Build history of the part. All positions in model axes, mm. A direction names the side the tool comes from. Round coordinates to 2 decimals unless told otherwise and drop trailing zeros. Write each loop counter-clockwise with the first axis right and the second up, starting at its lowest first coordinate (ties: lowest second). Pieces come first, ordered by that corner, then holes. Notation, with made-up numbers: (36.5, 28.5) -> (89.5, 28.5) arc R18 cw to (89.5, 38.5) -> close; hole circle Ø7 at (6.5, 3). An arc over 180 degrees is marked (long way). Answer in a Markdown table with one row per item. Add a question column.
from build123d import *

# Parameters (mm, degrees)
SKETCH1_R                = 88
BOSS_EXTRUDE3_DEPTH      = 25
SKETCH4_W                = 10.4719
SKETCH4_H                = 13.351164338
BOSS_EXTRUDE4_DEPTH      = 25
FILLET2_R                = 4
CIRPATTERN1_COUNT        = 30
FILLET2_OF_CIRPATTERN1_R = 4
SKETCH6_R                = 10
BOSS_EXTRUDE5_DEPTH      = 60
BOSS_EXTRUDE6_START      = 10
SKETCH7_R                = 10
BOSS_EXTRUDE6_DEPTH      = 10
SKETCH8_R                = 10
BOSS_EXTRUDE7_DEPTH      = 10
SKETCH9_R                = 10
BOSS_EXTRUDE8_DEPTH      = 25
SKETCH10_R               = 10
BOSS_EXTRUDE9_DEPTH      = 42.5
SKETCH12_R               = 12.5
CUT_EXTRUDE1_DEPTH       = 12
CUT_EXTRUDE2_START       = -55.5
SKETCH13_R               = 10
CUT_EXTRUDE2_DEPTH       = 55.5
SKETCH14_R               = 10
BOSS_EXTRUDE10_DEPTH     = 440
SKETCH15_R               = 105
BOSS_EXTRUDE12_DEPTH     = 25
BOSS_EXTRUDE13_START     = 30
SKETCH16_R               = 105
BOSS_EXTRUDE13_DEPTH     = 30
SKETCH17_R               = 10
BOSS_EXTRUDE14_DEPTH     = 50
SKETCH18_R               = 10
BOSS_EXTRUDE15_DEPTH     = 30
SKETCH19_R               = 105
SKETCH19_R_2             = 90
CUT_EXTRUDE3_DEPTH       = 100
SHELL3_START             = -30
SHELL3_OUTLINE_R         = 80
SHELL3_DEPTH             = 45
SCALE2_SCALE             = 0.2


# Read off the part's stored shape, not the designer's step: Shell3
with BuildPart() as part:
    # Sketch1 → Boss-Extrude3 (new body)
    with BuildSketch(Plane.XY):
        Circle(SKETCH1_R)
    extrude(amount=BOSS_EXTRUDE3_DEPTH)

    # Sketch4 → Boss-Extrude4 (add)
    with BuildSketch(Plane.XY.offset(25)):
        with Locations((0, 93.324417831)):
            Rectangle(SKETCH4_W, SKETCH4_H)
    boss_extrude4 = extrude(amount=-BOSS_EXTRUDE4_DEPTH)

    # Fillet2
    fillet2_edges = [part.edges().sort_by_distance(p)[0] for p in [
        (5.23595, 100, 12.5),
        (0, 100, 0),
        (-5.23595, 100, 12.5),
        (0, 100, 25),
    ]]
    fillet(fillet2_edges, radius=FILLET2_R)

    # CirPattern1: Boss-Extrude4 ×30 about axis
    cirpattern1_axis = Axis((0, 0.317667884, 0), (0, 0, 1))
    for i in range(1, CIRPATTERN1_COUNT):
        add(boss_extrude4.rotate(cirpattern1_axis, i * 360 / CIRPATTERN1_COUNT))

    # Fillet2 of CirPattern1
    fillet2_of_cirpattern1_edges = [part.edges().sort_by_distance(p)[0] for p in [
        (-15.603590285, 98.910317096, 12.5),
        (-20.725122215, 97.821701879, 0),
        (-25.846654145, 96.733086661, 12.5),
        (-20.725122215, 97.821701879, 25),
        (-35.7611788, 93.511662322, 12.5),
        (-40.544457139, 91.382009596, 0),
        (-45.327735478, 89.252356869, 12.5),
        (-40.544457139, 91.382009596, 25),
        (-54.3558322, 84.039982796, 12.5),
        (-58.591804732, 80.962368605, 0),
        (-62.827777264, 77.884754413, 12.5),
        (-58.591804732, 80.962368605, 25),
        (-70.574874905, 70.909236365, 12.5),
        (-74.078409304, 67.018167216, 0),
        (-77.581943702, 63.127098067, 12.5),
        (-74.078409304, 67.018167216, 25),
        (-83.709456921, 54.693299655, 12.5),
        (-86.327431921, 50.158833942, 0),
        (-88.945406921, 45.624368229, 12.5),
        (-86.327431921, 50.158833942, 25),
        (-93.185533987, 36.100886913, 12.5),
        (-94.803531519, 31.121202547, 0),
        (-96.42152905, 26.14151818, 12.5),
        (-94.803531519, 31.121202547, 25),
        (-98.588956064, 15.944575793, 12.5),
        (-99.136261871, 10.737308875, 0),
        (-99.683567678, 5.530041957, 12.5),
        (-99.136261871, 10.737308875, 25),
        (-99.683567678, -4.894706189, 12.5),
        (-99.136261871, -10.101973107, 0),
        (-98.588956064, -15.309240025, 12.5),
        (-99.136261871, -10.101973107, 25),
        (-96.42152905, -25.506182413, 12.5),
        (-94.803531519, -30.485866779, 0),
        (-93.185533987, -35.465551145, 12.5),
        (-94.803531519, -30.485866779, 25),
        (-88.945406921, -44.989032461, 12.5),
        (-86.327431921, -49.523498174, 0),
        (-83.709456921, -54.057963887, 12.5),
        (-86.327431921, -49.523498174, 25),
        (-77.581943702, -62.491762299, 12.5),
        (-74.078409304, -66.382831448, 0),
        (-70.574874905, -70.273900597, 12.5),
        (-74.078409304, -66.382831448, 25),
        (-62.827777264, -77.249418645, 12.5),
        (-58.591804732, -80.327032837, 0),
        (-54.3558322, -83.404647029, 12.5),
        (-58.591804732, -80.327032837, 25),
        (-45.327735478, -88.617021102, 12.5),
        (-40.544457139, -90.746673828, 0),
        (-35.7611788, -92.876326554, 12.5),
        (-40.544457139, -90.746673828, 25),
        (-25.846654145, -96.097750894, 12.5),
        (-20.725122215, -97.186366111, 0),
        (-15.603590285, -98.274981329, 12.5),
        (-20.725122215, -97.186366111, 25),
        (-5.23595, -99.364664232, 12.5),
        (0, -99.364664232, 0),
        (5.23595, -99.364664232, 12.5),
        (0, -99.364664232, 25),
        (15.603590285, -98.274981329, 12.5),
        (20.725122215, -97.186366111, 0),
        (25.846654145, -96.097750894, 12.5),
        (20.725122215, -97.186366111, 25),
        (35.7611788, -92.876326554, 12.5),
        (40.544457139, -90.746673828, 0),
        (45.327735478, -88.617021102, 12.5),
        (40.544457139, -90.746673828, 25),
        (54.3558322, -83.404647029, 12.5),
        (58.591804732, -80.327032837, 0),
        (62.827777264, -77.249418645, 12.5),
        (58.591804732, -80.327032837, 25),
        (70.574874905, -70.273900597, 12.5),
        (74.078409304, -66.382831448, 0),
        (77.581943702, -62.491762299, 12.5),
        (74.078409304, -66.382831448, 25),
        (83.709456921, -54.057963887, 12.5),
        (86.327431921, -49.523498174, 0),
        (88.945406921, -44.989032461, 12.5),
        (86.327431921, -49.523498174, 25),
        (93.185533987, -35.465551145, 12.5),
        (94.803531519, -30.485866779, 0),
        (96.42152905, -25.506182413, 12.5),
        (94.803531519, -30.485866779, 25),
        (98.588956064, -15.309240025, 12.5),
        (99.136261871, -10.101973107, 0),
        (99.683567678, -4.894706189, 12.5),
        (99.136261871, -10.101973107, 25),
        (99.683567678, 5.530041957, 12.5),
        (99.136261871, 10.737308875, 0),
        (98.588956064, 15.944575793, 12.5),
        (99.136261871, 10.737308875, 25),
        (96.42152905, 26.14151818, 12.5),
        (94.803531519, 31.121202547, 0),
        (93.185533987, 36.100886913, 12.5),
        (94.803531519, 31.121202547, 25),
        (88.945406921, 45.624368229, 12.5),
        (86.327431921, 50.158833942, 0),
        (83.709456921, 54.693299655, 12.5),
        (86.327431921, 50.158833942, 25),
        (77.581943702, 63.127098067, 12.5),
        (74.078409304, 67.018167216, 0),
        (70.574874905, 70.909236365, 12.5),
        (74.078409304, 67.018167216, 25),
        (62.827777264, 77.884754413, 12.5),
        (58.591804732, 80.962368605, 0),
        (54.3558322, 84.039982796, 12.5),
        (58.591804732, 80.962368605, 25),
        (45.327735478, 89.252356869, 12.5),
        (40.544457139, 91.382009596, 0),
        (35.7611788, 93.511662322, 12.5),
        (40.544457139, 91.382009596, 25),
        (25.846654145, 96.733086661, 12.5),
        (20.725122215, 97.821701879, 0),
        (15.603590285, 98.910317096, 12.5),
        (20.725122215, 97.821701879, 25),
    ]]
    fillet(fillet2_of_cirpattern1_edges, radius=FILLET2_OF_CIRPATTERN1_R)

    # Sketch6 → Boss-Extrude5 (add)
    with BuildSketch(Plane.XY.offset(25)):
        Circle(SKETCH6_R)
    extrude(amount=BOSS_EXTRUDE5_DEPTH)

    # Sketch7 → Boss-Extrude6 (add)
    with BuildSketch(Plane(origin=(0, 0, 0), x_dir=(-1, 0, 0), z_dir=(0, 0, -1)).offset(BOSS_EXTRUDE6_START)):
        with Locations(Location((0, 0, 0), (0, 0, 180))):
            Circle(SKETCH7_R)
    extrude(amount=-BOSS_EXTRUDE6_DEPTH)

    # Sketch8 → Boss-Extrude7 (add)
    with BuildSketch(Plane.XY.offset(85)):
        Circle(SKETCH8_R)
    extrude(amount=BOSS_EXTRUDE7_DEPTH)

    # Sketch9 → Boss-Extrude8 (add)
    with BuildSketch(Plane.XY.offset(95)):
        Circle(SKETCH9_R)
    extrude(amount=BOSS_EXTRUDE8_DEPTH)

    # Sketch10 → Boss-Extrude9 (add)
    with BuildSketch(Plane.XY.offset(120)):
        Circle(SKETCH10_R)
    extrude(amount=BOSS_EXTRUDE9_DEPTH)

    # Sketch12 → Cut-Extrude1 (cut)
    with BuildSketch(Plane.XY.offset(162.5)):
        Circle(SKETCH12_R)
    extrude(amount=-CUT_EXTRUDE1_DEPTH, mode=Mode.SUBTRACT)

    # Sketch13 → Cut-Extrude2 (cut)
    with BuildSketch(Plane.XY.offset(150.5).offset(CUT_EXTRUDE2_START)):
        Circle(SKETCH13_R)
    extrude(amount=CUT_EXTRUDE2_DEPTH, mode=Mode.SUBTRACT)

    # Sketch14 → Boss-Extrude10 (add)
    with BuildSketch(Plane.XY.offset(95)):
        Circle(SKETCH14_R)
    extrude(amount=BOSS_EXTRUDE10_DEPTH)

    # Sketch15 → Boss-Extrude12 (add)
    with BuildSketch(Plane(origin=(0, 0, 0), x_dir=(-1, 0, 0), z_dir=(0, 0, -1))):
        Circle(SKETCH15_R)
    extrude(amount=-BOSS_EXTRUDE12_DEPTH)

    # Sketch16 → Boss-Extrude13 (add)
    with BuildSketch(Plane(origin=(0, 0, 0), x_dir=(-1, 0, 0), z_dir=(0, 0, -1)).offset(BOSS_EXTRUDE13_START)):
        Circle(SKETCH16_R)
    extrude(amount=-BOSS_EXTRUDE13_DEPTH)

    # Sketch17 → Boss-Extrude14 (add)
    with BuildSketch(Plane.XY.offset(535)):
        Circle(SKETCH17_R)
    extrude(amount=BOSS_EXTRUDE14_DEPTH)

    # Sketch18 → Boss-Extrude15 (add)
    with BuildSketch(Plane.XY.offset(585)):
        Circle(SKETCH18_R)
    extrude(amount=BOSS_EXTRUDE15_DEPTH)

    # Sketch19 → Cut-Extrude3 (cut)
    with BuildSketch(Plane(origin=(0, 0, -30), x_dir=(-1, 0, 0), z_dir=(0, 0, -1))):
        Circle(SKETCH19_R)
        Circle(SKETCH19_R_2, mode=Mode.SUBTRACT)
    extrude(amount=-CUT_EXTRUDE3_DEPTH, mode=Mode.SUBTRACT)

    # Shell3 outline → Shell3 (cut)
    with BuildSketch(Plane.XY.offset(SHELL3_START)):
        Circle(SHELL3_OUTLINE_R)
    extrude(amount=SHELL3_DEPTH, mode=Mode.SUBTRACT)


with BuildPart() as part_1:
    # Scale2: scaled about (0, 0, 92.038106236)
    add(part.part.scale(SCALE2_SCALE).moved(Location((0, 0, 73.630484989))))


solid = part_1.part
(1) Mould opens along Y. For faces 1 (the face through (12, -11, 67.63)), 2 (the face through (-3.47, -15.62, 72.07)), 3 (the face through (2.343, 17.847, 73.053)) say: pulls with the +Y half, pulls with the -Y half, needs draft (parallel to the pull), parting line crosses it, or undercut.
(2) Saw through at C-C (z = 90). List the corners of the cut face in (x, y).
(3) Probe line 1 along Y through (x, z) = (0, 71.5); line 2 along Z through (x, y) = (2, -3); line 3 along Z through (x, y) = (16, 4). List the from-to ranges inside material, lowest first.
(4) Saw through at D-D (y = -6). List the corners of the cut face in (x, z), plus the area to 3 significant figures.
(5) Saw through at A-A (x = 0). List the corners of the cut face in (y, z), plus the area to 3 significant figures.
(6) Drop flat-ended pins along their axis: P1, Ø12, axis at x = -11.5, y = 9, coming from the +Z side; P2, Ø10, axis at y = -1.5, z = 82.5, coming from the +X side; P3, Ø6, axis at x = -7, y = 0, coming from the -Z side; P4, Ø1.5, axis at y = 0, z = 117, coming from the +X side. Give the stop position or say it passes through.
(7) Which spindle directions (+Z, -Z, +X, -X, +Y, -Y) get a long thin tool onto all of the face, cutting with end or side? Do faces 4 (the face through (0, 0, 196.63)), 5 (the face through (0, 0, 76.63)), 6 (the face through (0, -2, 137)). Say none if no direction does.
Answer sheet:
| question | item | result |
|---|---|---|
| 1 | face 1 | needs draft |
| 1 | face 2 | undercut |
| 1 | face 3 | parting line crosses it |
| 2 | outline | circle Ø4 at (0, 0) |
| 3 | line 1 | y = -18 to -16, 16 to 18 |
| 3 | line 2 | z = 76.63 to 78.63 |
| 3 | line 3 | z = 67.63 to 78.63 |
| 4 | outline | (-16.97, 67.63) -> (-14.83, 67.63) -> (-14.83, 76.63) -> (14.83, 76.63) -> (14.83, 67.63) -> (16.97, 67.63) -> (16.97, 78.63) -> (-16.97, 78.63) -> close |
| 4 | area | 106 mm² |
| 5 | outline | (-18, 67.63) -> (-16, 67.63) -> (-16, 76.63) -> (16, 76.63) -> (16, 67.63) -> (18, 67.63) -> (18, 78.63) -> (2, 78.63) -> (2, 196.63) -> (-2, 196.63) -> (-2, 78.63) -> (-18, 78.63) -> close |
| 5 | area | 580 mm² |
| 6 | P1 | stops at z = 78.63 |
| 6 | P2 | stops at x = 18 |
| 6 | P3 | stops at z = 76.63 |
| 6 | P4 | stops at x = 2 |
| 7 | face 4 | +Z, +X, -X, +Y, -Y |
| 7 | face 5 | -Z |
| 7 | face 6 | +Z |
